Check sheet for the drawn part. Datum: minimum x, y, z corner. Units: mm. A direction names the side the tool comes from. Round coordinates to 2 decimals unless told otherwise and drop trailing zeros. Order: outer loops, then holes, each group sorted by start corner. A loop starts at its lowest first (then second) coordinate and runs counter-clockwise, first axis right, second up. Notation, with made-up numbers: (77, 10.5) -> (115, 10.5) arc R17 ccw to (115, 35.5) -> close; hole circle Ø9 at (73, 13.25). An arc over 180 degrees is marked (long way). Answer as a JSON object with one key per item and string values. Group by question number.
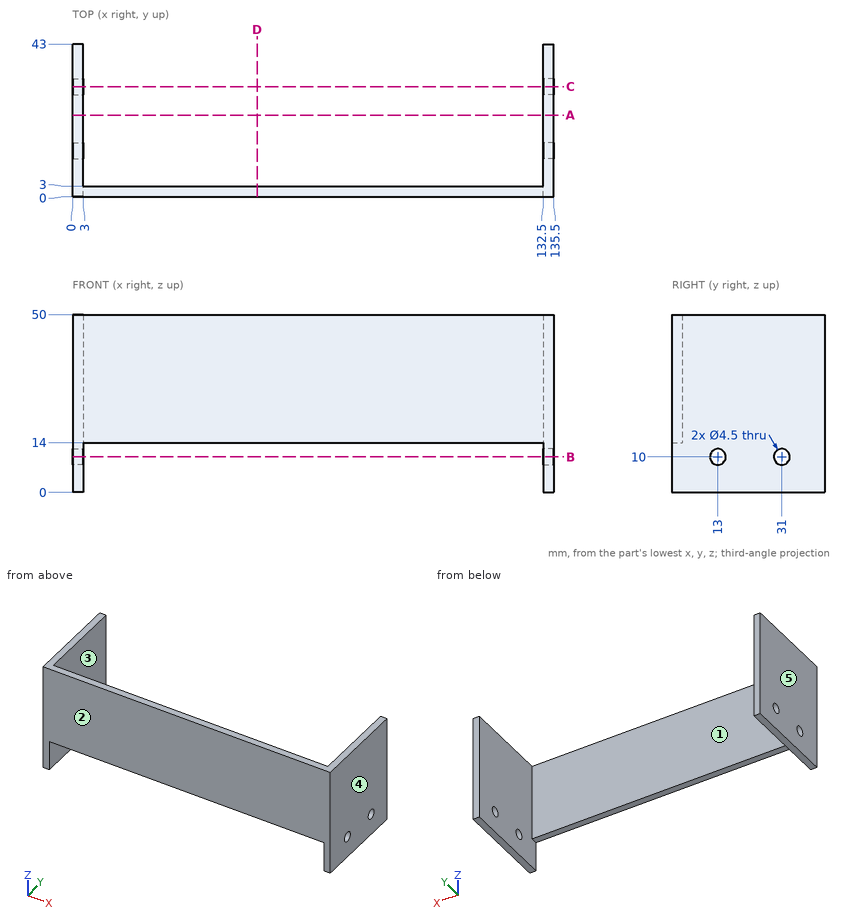
Item 1: Set-up check for the marked faces 1 and 2: record each of +Z, -Z, +X, -X, +Y, -Y from which the full face is reachable in a straight line by a thin tool's end or side.
Item 2: Sectioned sample at D-D, the plane x = 52. Enter the section's corners in (y, z), then the cut area to 3 significant figures.
Item 3: Thickness scan on L1, parallel to X at y = 26.5, z = 42; L2, parallel to Y at x = 134.45, z = 10; L3, parallel to Y at x = 22, z = 32.5. Record the ranges inside material, lowest first.
Item 4: Depth check by flat-ended pin: pin 1 Ø4 at (x, z) = (23, 13.5) entering from -Y; pin 2 Ø3.5 at (x, y) = (39, 1) entering from -Z; pin 3 Ø10 at (x, z) = (105, 43) entering from +Y; pin 4 Ø4 at (y, z) = (31, 10) entering from +X. Enter the tip coordinate at first touch or a pass-through.
Item 5: Sectioned sample at A-A, the plane y = 23. Enter the section's corners in (x, z), then the cut area to 3 significant figures.
Item 6: Mould release check, pull along X, two halves, no side actions. Record for the marked faces 3, 4 and 5: pulls with the +X half, pulls with the -X half, needs draft (parallel to the pull), parting line crosses it, or undercut.
Item 7: Sectioned sample at B-B, the plane z = 10. Enter the section's corners in (x, y), then the cut area to 3 significant figures.
Item 8: Sectioned sample at C-C, the plane y = 31. Enter the section's corners in (x, z).
Result:
{
 "1": {"face 1": "+Z, -Z, +Y", "face 2": "+Z, -Z, +X, -X, -Y"},
 "2": {"outline": "(0, 14) -> (3, 14) -> (3, 50) -> (0, 50) -> close", "area": "108 mm2"},
 "3": {"L1": "x = 0 to 3, 132.5 to 135.5", "L2": "y = 0 to 10.75, 15.25 to 28.75, 33.25 to 43", "L3": "y = 0 to 3"},
 "4": {"pin 1": "stops at y = 0", "pin 2": "stops at z = 14", "pin 3": "stops at y = 3", "pin 4": "passes through"},
 "5": {"outline": "(0, 0) -> (3, 0) -> (3, 50) -> (0, 50) -> close; (132.5, 0) -> (135.5, 0) -> (135.5, 50) -> (132.5, 50) -> close", "area": "300 mm2"},
 "6": {"face 3": "undercut", "face 4": "pulls with the +X half", "face 5": "pulls with the -X half"},
 "7": {"outline": "(0, 0) -> (3, 0) -> (3, 10.75) -> (0, 10.75) -> close; (0, 15.25) -> (3, 15.25) -> (3, 28.75) -> (0, 28.75) -> close; (0, 33.25) -> (3, 33.25) -> (3, 43) -> (0, 43) -> close; (132.5, 0) -> (135.5, 0) -> (135.5, 10.75) -> (132.5, 10.75) -> close; (132.5, 15.25) -> (135.5, 15.25) -> (135.5, 28.75) -> (132.5, 28.75) -> close; (132.5, 33.25) -> (135.5, 33.25) -> (135.5, 43) -> (132.5, 43) -> close", "area": "204 mm2"},
 "8": {"outline": "(0, 0) -> (3, 0) -> (3, 7.75) -> (0, 7.75) -> close; (0, 12.25) -> (3, 12.25) -> (3, 50) -> (0, 50) -> close; (132.5, 0) -> (135.5, 0) -> (135.5, 7.75) -> (132.5, 7.75) -> close; (132.5, 12.25) -> (135.5, 12.25) -> (135.5, 50) -> (132.5, 50) -> close"}
}
